Design review of the part shown in the three views and the two pictorial views. Dimensions are in mm from the part's minimum x, y and z. Coordinates: 2 decimals unless noted, no trailing zeros. Write each loop counter-clockwise with the first axis right and the second up, starting at its lowest first coordinate (ties: lowest second). Pieces come first, ordered by that corner, then holes. Notation, with made-up numbers: (60, 16.5) - (96, 16.5) arc R8 cw to (96, 31.5) - close; hole circle Ø7 at (75.25, 49). An arc over 180 degrees is marked (long way). Return JSON: item names as keys, results as strings. Group by question number.
(1) To check wall thickness, follow L1, parallel to Y at x = 5, z = 3.95; L2, parallel to Y at x = 14, z = 0.9; L3, parallel to X at y = 27.5, z = 0.5. State the ranges of each line that lie inside material, in increasing order. Write a range as from..to.
(2) We need section C-C on x = 83.5. State the section outline as (y, z) points.
(3) We need section A-A on y = 41. State the section outline as (x, z) points.
(4) We need section D-D on x = 45. State the section outline as (y, z) points, then the cut area to 3 significant figures.
(5) We need section B-B on z = 1.7. State the section outline as (x, y) points.
(6) For pin 1 Ø3 at (x, z) = (61.5, 1.5) entering from +Y; pin 2 Ø1 at (x, z) = (14.5, 3) entering from +Y, all flat-tipped, find the tip position at first contact; note any pin that passes through.
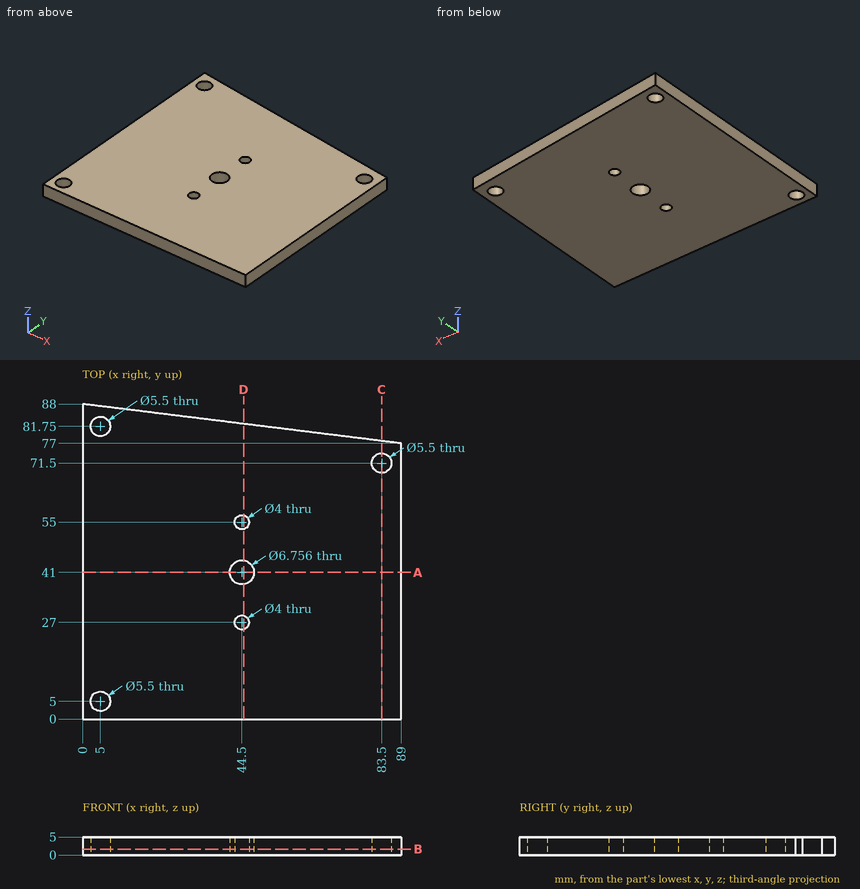
Ans:
{
 "1": {"L1": "0..2.25, 7.75..79, 84.5..87.38", "L2": "0..86.27", "L3": "0..42.56, 46.44..89"},
 "2": {"outline": "(0, 0) - (68.75, 0) - (68.75, 5) - (0, 5) - close; (74.25, 0) - (77.68, 0) - (77.68, 5) - (74.25, 5) - close"},
 "3": {"outline": "(0, 0) - (41.12, 0) - (41.12, 5) - (0, 5) - close; (47.88, 0) - (89, 0) - (89, 5) - (47.88, 5) - close"},
 "4": {"outline": "(0, 0) - (25.06, 0) - (25.06, 5) - (0, 5) - close; (28.94, 0) - (37.66, 0) - (37.66, 5) - (28.94, 5) - close; (44.34, 0) - (53.06, 0) - (53.06, 5) - (44.34, 5) - close; (56.94, 0) - (82.44, 0) - (82.44, 5) - (56.94, 5) - close", "area": "340 mm²"},
 "5": {"outline": "(0, 0) - (89, 0) - (89, 77) - (0, 88) - close; hole circle Ø5.5 at (5, 5); hole circle Ø5.5 at (5, 81.75); hole circle Ø6.76 at (44.5, 41); hole circle Ø4 at (44.5, 27); hole circle Ø4 at (44.5, 55); hole circle Ø5.5 at (83.5, 71.5)"},
 "6": {"pin 1": "y = 80.58", "pin 2": "y = 86.27"}
}
